Part model, mm, in its own coordinate system. Face numbers are marked on the shaded views. A direction names the side the tool comes from. Round coordinates to 2 decimals unless told otherwise and drop trailing zeros. Loops run counter-clockwise (first coordinate to the right, second up) from the corner with the lowest first, then second, coordinate; pieces in that order, holes last.
from build123d import *

# Parameters (mm, degrees)
F0_R     = 14.2875
F1_DEPTH = 31.75
F2_DEPTH = 4.7625
F3_R     = 5.5626
F4_DEPTH = 4.7752
F5_DEPTH = 15.875
F6_DEPTH = 15.875


with BuildPart() as f1:
    # F0 (on Front) → F1 (new body, symmetric)
    with BuildSketch(Plane.XZ):
        with BuildLine():
            ThreePointArc((0, 19.05), (12.2967221242, 14.5496778315), (18.7835533113, 3.175))
            Line((18.7835533113, 3.175), (27.86051193, 3.175))
            Line((27.86051193, 3.175), (69.85, 3.175))
            Line((69.85, 3.175), (96.8502, 3.175))
            Line((96.8502, 3.175), (96.8502, 19.05))
            Line((96.8502, 19.05), (0, 19.05))
        make_face()
        with BuildLine():
            ThreePointArc((18.57367462, -4.2333333333), (18.930544122, -2.1300232967), (19.05, 0))
            ThreePointArc((19.05, 0), (18.9832714591, 1.5930802583), (18.7835533113, 3.175))
            ThreePointArc((18.7835533113, 3.175), (12.2967221242, 14.5496778315), (0, 19.05))
            ThreePointArc((0, 19.05), (-18.8046153549, -3.0477764606), (6.0170355936, -18.07478306))
            ThreePointArc((6.0170355936, -18.07478306), (14.1092944486, -12.7996214852), (18.57367462, -4.2333333333))
        make_face()
        Circle(F0_R, mode=Mode.SUBTRACT)
        with BuildLine():
            ThreePointArc((18.7835533113, 3.175), (18.9832714591, 1.5930802583), (19.05, 0))
            ThreePointArc((19.05, 0), (18.930544122, -2.1300232967), (18.57367462, -4.2333333333))
            ThreePointArc((18.57367462, -4.2333333333), (21.9206308285, 1.0960350187), (27.86051193, 3.175))
            Line((27.86051193, 3.175), (18.7835533113, 3.175))
        make_face()
    extrude(amount=F1_DEPTH, both=True)

    # F0 (on Front) → F2 (join, symmetric)
    with BuildSketch(Plane.XZ):
        with BuildLine():
            ThreePointArc((27.86051193, 3.175), (21.9206308285, 1.0960350187), (18.57367462, -4.2333333333))
            ThreePointArc((18.57367462, -4.2333333333), (14.1092944486, -12.7996214852), (6.0170355936, -18.07478306))
            Line((6.0170355936, -18.07478306), (69.85, 3.175))
            Line((69.85, 3.175), (27.86051193, 3.175))
        make_face()
    extrude(amount=F2_DEPTH, both=True)

    # F3 (on face) → F4 (join)
    with BuildSketch(Plane.XY.offset(19.05)):
        with BuildLine():
            ThreePointArc((47.3970452561, -31.75), (50.6840471289, -31.3172579939), (53.7470452561, -30.0485226281))
            Line((53.7470452561, -30.0485226281), (92.3789934298, -7.7443569506))
            ThreePointArc((92.3789934298, -7.7443569506), (95.652143832, -4.4712065327), (96.8502, 8.65e-08))
            ThreePointArc((96.8502, 8.65e-08), (95.6521437887, 4.4712066076), (92.3789934298, 7.7443569506))
            Line((92.3789934298, 7.7443569506), (53.7470452561, 30.0485226281))
            ThreePointArc((53.7470452561, 30.0485226281), (50.6840471289, 31.3172579939), (47.3970452561, 31.75))
            ThreePointArc((47.3970452561, 31.75), (38.4167891351, 28.0302561211), (34.6970452561, 19.05))
            Line((34.6970452561, 19.05), (34.6970452561, -19.05))
            ThreePointArc((34.6970452561, -19.05), (38.4167891351, -28.0302561211), (47.3970452561, -31.75))
        make_face()
        with Locations((50.8, -19.05)):
            Circle(F3_R, mode=Mode.SUBTRACT)
        with Locations((84.1502, 0)):
            Circle(F3_R, mode=Mode.SUBTRACT)
        with Locations((50.8, 19.05)):
            Circle(F3_R, mode=Mode.SUBTRACT)
    extrude(amount=F4_DEPTH)

    # F3 (on face) → F5 (cut, through all)
    with BuildSketch(Plane.XY.offset(19.05)):
        Polygon((53.7470452561, -30.0485226281), (50.8, -31.75), (96.8502, -31.75), (96.8502, -5.1629046338), (92.3789934298, -7.7443569506), align=None)
        Polygon((53.7470452561, 30.0485226281), (92.3789934298, 7.7443569506), (96.8502, 5.1629046338), (96.8502, 31.75), (50.8, 31.75), align=None)
        with BuildLine():
            ThreePointArc((92.3789934298, 7.7443569506), (95.6521437887, 4.4712066076), (96.8502, 8.65e-08))
            Line((96.8502, 8.65e-08), (96.8502, 5.1629046338))
            Line((96.8502, 5.1629046338), (92.3789934298, 7.7443569506))
        make_face()
        with BuildLine():
            ThreePointArc((96.8502, 8.65e-08), (95.652143832, -4.4712065327), (92.3789934298, -7.7443569506))
            Line((92.3789934298, -7.7443569506), (96.8502, -5.1629046338))
            Line((96.8502, -5.1629046338), (96.8502, 8.65e-08))
        make_face()
    extrude(amount=-F5_DEPTH, mode=Mode.SUBTRACT)

    # F3 (on face) → F6 (cut, through all)
    with BuildSketch(Plane.XY.offset(19.05)):
        with Locations((84.1502, 0)):
            Circle(F3_R)
        with Locations((50.8, 19.05)):
            Circle(F3_R)
        with Locations((50.8, -19.05)):
            Circle(F3_R)
    extrude(amount=-F6_DEPTH, mode=Mode.SUBTRACT)


solid = f1.part
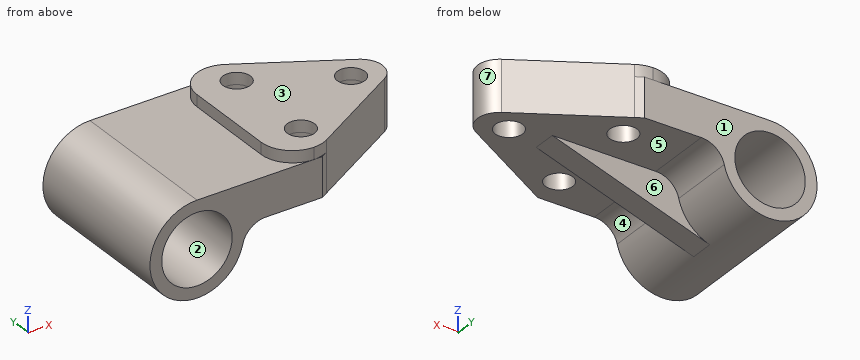
1) Slice it at D-D, the plane z = 0. Give the cut face in (x, y).
Values:
outline: (-19.05, -31.75) - (-14.29, -31.75) - (-14.29, 31.75) - (-19.05, 31.75) - close; (14.29, -31.75) - (20.76, -31.75) - (20.76, -4.76) - (60.31, -4.76) - (60.31, 4.76) - (20.76, 4.76) - (20.76, 31.75) - (14.29, 31.75) - close
2) Mould opens along Z. For the marked faces 1, 2, 3 and 4 say: released by +Z, released by -Z, zero draft, split by the parting line, or undercut.
Values:
face 1: zero draft
face 2: undercut
face 3: released by +Z
face 4: released by -Z
3) Slice it at B-B, the plane z = 12. Give the cut face in (x, y).
Values:
outline: (-14.8, -31.75) - (-7.75, -31.75) - (-7.75, 31.75) - (-14.8, 31.75) - close; (7.75, -31.75) - (50.8, -31.75) - (92.38, -7.74) arc R8.94 ccw to (92.38, 7.74) - (50.8, 31.75) - (7.75, 31.75) - close; hole circle Ø11.13 at (50.8, -19.05); hole circle Ø11.13 at (50.8, 19.05); hole circle Ø11.13 at (84.15, 0)
4) Drop flat-ended pins along their axis: pin 1 Ø3 at (y, z) = (-5, 10.5) entering from +X; pin 2 Ø17 at (x, z) = (0, 0) entering from +Y; pin 3 Ø18 at (x, y) = (84.15, 0) entering from -Z (3 decimals); pin 4 Ø1 at (y, z) = (21.5, 16) entering from +X. Give the stop position or say it passes through.
Values:
pin 1: stops at x = 96.14
pin 2: passes through
pin 3: stops at z = 3.175
pin 4: stops at x = 69.42
5) Wall check: line 1 along X through (y, z) = (19, 13); line 2 along X through (y, z) = (24, 5); line 3 along Y through (x, z) = (50.8, 21.35). Give the ranges that are in metal, low to high.
Values:
line 1: x = -13.92 to -5.93, 5.93 to 45.24, 56.36 to 72.88
line 2: x = -18.38 to -13.38, 13.38 to 48.26, 53.34 to 64.22
line 3: y = -31.29 to -24.61, -13.49 to 13.49, 24.61 to 31.29
6) Tool access for the marked faces 5, 6 and 7: list every direction of +Z, -Z, +X, -X, +Y, -Y with a clear straight run to the whole face (end or side of a thin tool).
Values:
face 5: -Z, +X
face 6: -Z, +X, +Y
face 7: +Z, -Z, +X
7) Slice it at A-A, the plane y = 0. Give the number of separate pieces and of enclosed holes in the cut face, then the cut area to 3 significant figures.
Values:
separate pieces: 2
enclosed holes: 1
area: 2,340 mm2
